The model under review builds one solid part; all positions refer to its coordinate system, in mm. A direction names the side the tool comes from. Coordinates: 2 decimals unless noted, no trailing zeros. Write each loop counter-clockwise with the first axis right and the second up, starting at its lowest first coordinate (ties: lowest second). Pieces come first, ordered by that corner, then holes.
1) For line 1 (Z direction, x = -23, y = -16.25); line 2 (Y direction, x = -11.25, z = -1.3); line 3 (Y direction, x = -28.25, z = -1.4), list the stretches that pass through material, from the lowest coordinate up.
2) Add section C-C, the plane y = -11.5. State the section outline as (x, z) points.
3) Add section B-B, the plane x = -22.25. State the section outline as (y, z) points.
4) Add section A-A, the plane y = -16.5. State the section outline as (x, z) points, then the cut area to 3 significant figures.
5) Machinability: for faces 1 (the flat face through (-29.212, -13, -1)), 2 (the flat face through (-28, -14.861, -2)), which of the approach directions +Z, -Z, +X, -X, +Y, -Y give a long, thin tool a straight path to every point of the face, cutting with its end or side? Answer none if there is none.
6) For P1, Ø1, axis at x = -12, y = -15.5, coming from the -Z side, flat-tipped, find the tip position at first contact; note if it passes through.
from build123d import *

# Parameters (mm, degrees)
SKETCH1_W           = 19.981739869
SKETCH1_H           = 10.800167474
BOSS_EXTRUDE1_DEPTH = 1.5
SKETCH3_W           = 2.678049678
SKETCH3_H           = 6.088868787
BOSS_EXTRUDE2_DEPTH = 1.920000865
FILLET1_R           = 1.5
FILLET2_R           = 0.25


with BuildPart() as part:
    # Sketch1 → Boss-Extrude1 (new body)
    with BuildSketch(Plane.XY):
        with Locations((-19.22144379, -14.172432084)):
            Rectangle(SKETCH1_W, SKETCH1_H)
    extrude(amount=-BOSS_EXTRUDE1_DEPTH)

    # Sketch3 → Boss-Extrude2 (add)
    with BuildSketch(Plane(origin=(0, 0, -1.5), x_dir=(-1, 0, 0), z_dir=(0, 0, -1))):
        with Locations((27.873288885, -11.816782741)):
            Rectangle(SKETCH3_W, SKETCH3_H)
    extrude(amount=BOSS_EXTRUDE2_DEPTH)

    # Fillet1
    fillet1_edges = [part.edges().sort_by_distance(p)[0] for p in [
        (-26.534264046, -11.81678274, -1.5),
    ]]
    fillet(fillet1_edges, radius=FILLET1_R)

    # Fillet2
    fillet2_edges = [part.edges().sort_by_distance(p)[0] for p in [
        (-26.534264046, -14.861217134, -3.210000433),
        (-26.534264046, -11.81678274, -3.420000865),
        (-26.534264046, -8.772348347, -3.210000433),
        (-19.221443789, -19.572515821, -1.5),
        (-26.094924218, -14.861217134, -1.939339828),
        (-26.094924218, -8.772348347, -1.939339828),
        (-9.230573855, -14.172432084, -1.5),
        (-17.13241895, -8.772348347, -1.5),
    ]]
    fillet(fillet2_edges, radius=FILLET2_R)


solid = part.part
Geometry results:
1. line 1: z = -1.5 to 0
1. line 2: y = -19.57 to -8.78
1. line 3: y = -19.52 to -8.77
2. outline: (-29.21, -3.42) - (-26.78, -3.42) arc R0.25 ccw to (-26.53, -3.17) - (-26.53, -3) arc R1.5 cw to (-25.03, -1.5) - (-9.48, -1.5) arc R0.25 ccw to (-9.23, -1.25) - (-9.23, 0) - (-29.21, 0) - close
3. outline: (-19.57, -1.25) arc R0.25 ccw to (-19.32, -1.5) - (-9.02, -1.5) arc R0.25 ccw to (-8.77, -1.25) - (-8.77, 0) - (-19.57, 0) - close
4. outline: (-29.21, -1.5) - (-9.48, -1.5) arc R0.25 ccw to (-9.23, -1.25) - (-9.23, 0) - (-29.21, 0) - close
4. area: 30.0 mm2
5. face 1: +Z, -Z, -X, +Y, -Y
5. face 2: -Z, +X, -X, -Y
6. P1: stops at z = -1.5
